The model under review builds one solid part; all positions refer to its coordinate system, in mm. A direction names the side the tool comes from. Give positions to 0.01 mm unless a question says otherwise; leave off trailing zeros. Order: outer loops, then holes, each group sorted by start corner. A loop starts at its lowest first (then second) coordinate and runs counter-clockwise, first axis right, second up.
```python
from build123d import *

# Parameters (mm, degrees)
BOSS_EXTRUDE1_DEPTH = 8
SKETCH4_W           = 10
SKETCH4_H           = 4
SKETCH4_W_2         = 4
SKETCH4_H_2         = 10
BOSS_EXTRUDE2_DEPTH = 14
SKETCH5_R           = 1
CUT_EXTRUDE1_DEPTH  = 16
SKETCH6_R           = 1
CUT_EXTRUDE2_DEPTH  = 16
FILLET1_R           = 2


with BuildPart() as part:
    # Sketch3 → Boss-Extrude1 (new body)
    with BuildSketch(Plane(origin=(0, 0, 0), x_dir=(1, 0, 0), z_dir=(0, 1, 0))):
        with BuildLine():
            Line((-40, 25), (40, 25))
            ThreePointArc((40, 25), (47.071067812, 22.071067812), (50, 15))
            Line((50, 15), (50, -15))
            ThreePointArc((50, -15), (47.071067812, -22.071067812), (40, -25))
            Line((40, -25), (-40, -25))
            ThreePointArc((-40, -25), (-47.071067812, -22.071067812), (-50, -15))
            Line((-50, -15), (-50, 15))
            ThreePointArc((-50, 15), (-47.071067812, 22.071067812), (-40, 25))
        make_face()
    extrude(amount=BOSS_EXTRUDE1_DEPTH)

    # Sketch4 → Boss-Extrude2 (add)
    with BuildSketch(Plane(origin=(0, 8, 0), x_dir=(1, 0, 0), z_dir=(0, 1, 0))):
        with Locations((-25, 20)):
            Rectangle(SKETCH4_W, SKETCH4_H)
        with Locations((-25, 8)):
            Rectangle(SKETCH4_W, SKETCH4_H)
        with Locations((-6, -9)):
            Rectangle(SKETCH4_W_2, SKETCH4_H_2)
        with Locations((6, -9)):
            Rectangle(SKETCH4_W_2, SKETCH4_H_2)
        with Locations((25, 8)):
            Rectangle(SKETCH4_W, SKETCH4_H)
        with Locations((25, 20)):
            Rectangle(SKETCH4_W, SKETCH4_H)
    extrude(amount=BOSS_EXTRUDE2_DEPTH)

    # Sketch5 → Cut-Extrude1 (cut)
    with BuildSketch(Plane.XY.offset(-6)):
        with Locations((-25, 18)):
            Circle(SKETCH5_R)
        with Locations((25, 18)):
            Circle(SKETCH5_R)
    extrude(amount=-CUT_EXTRUDE1_DEPTH, mode=Mode.SUBTRACT)

    # Sketch6 → Cut-Extrude2 (cut)
    with BuildSketch(Plane.ZY.offset(8)):
        with Locations((9, 18)):
            Circle(SKETCH6_R)
    extrude(amount=-CUT_EXTRUDE2_DEPTH, mode=Mode.SUBTRACT)

    # Fillet1
    fillet1_edges = [part.edges().sort_by_distance(p)[0] for p in [
        (47.071067812, 8, -22.071067812),
        (0, 8, -25),
        (-47.071067812, 8, -22.071067812),
        (-50, 8, 0),
        (-30, 22, -20),
        (-47.071067812, 8, 22.071067812),
        (-20, 22, -20),
        (0, 8, 25),
        (-30, 22, -8),
        (-20, 22, -8),
        (47.071067812, 8, 22.071067812),
        (-6, 22, 14),
        (-6, 22, 4),
        (6, 22, 4),
        (6, 22, 14),
        (30, 22, -8),
        (20, 22, -8),
        (30, 22, -20),
        (20, 22, -20),
        (50, 8, 0),
    ]]
    fillet(fillet1_edges, radius=FILLET1_R)


solid = part.part
```
Item 1: Take a section at A-A (z = 9). Give the boundary of the cut face in (x, y), and give its area (3 significant figures).
Values found:
outline: (-50, 0) - (50, 0) - (50, 6) arc R2 ccw to (48, 8) - (8, 8) - (8, 17) - (4, 17) - (4, 8) - (-4, 8) - (-4, 17) - (-8, 17) - (-8, 8) - (-48, 8) arc R2 ccw to (-50, 6) - close; (-8, 19) - (-4, 19) - (-4, 22) - (-8, 22) - close; (4, 19) - (8, 19) - (8, 22) - (4, 22) - close
area: 894 mm2
Item 2: For faces 1 (the flat face through (-30, 14, -8)), 2 (the flat face through (-25, 22, -8)), 3 (the flat face through (25, 15, -10)), 4 (the flat face through (20, 14, -8)), list the 3-axis set-ups (+Z, -Z, +X, -X, +Y, -Y) from which the entire face can be reached by the end or side of a thin tool; tool diameter is ignored.
Values found:
face 1: +Z, -Z, -X, +Y
face 2: +Z, -Z, +X, -X, +Y
face 3: +X, -X, +Y
face 4: +Z, -Z, +Y
Item 3: Draft analysis for pull direction Y (two halves, no side actions). For faces 5 (the flat face through (6, 22, 9)), 6 (the cylindrical face through (-25, 17, -8)), 7 (the flat face through (-6, 14, 4)), state which applies: released by +Y, released by -Y, zero draft, split by the parting line, or undercut.
Values found:
face 5: released by +Y
face 6: undercut
face 7: zero draft
Item 4: Take a section at C-C (y = 9.75). Give the boundary of the cut face in (x, z), and give its area (3 significant figures).
Values found:
outline: (-30, -22) - (-20, -22) - (-20, -18) - (-30, -18) - close; (-30, -10) - (-20, -10) - (-20, -6) - (-30, -6) - close; (-8, 4) - (-4, 4) - (-4, 14) - (-8, 14) - close; (4, 4) - (8, 4) - (8, 14) - (4, 14) - close; (20, -22) - (30, -22) - (30, -18) - (20, -18) - close; (20, -10) - (30, -10) - (30, -6) - (20, -6) - close
area: 240 mm2
Item 5: Take a section at B-B (x = -25). Give the boundary of the cut face in (y, z).
Values found:
outline: (0, -25) - (6, -25) arc R2 ccw to (8, -23) - (8, -22) - (17, -22) - (17, -18) - (8, -18) - (8, -10) - (17, -10) - (17, -6) - (8, -6) - (8, 23) arc R2 ccw to (6, 25) - (0, 25) - close; (19, -22) - (22, -22) - (22, -18) - (19, -18) - close; (19, -10) - (22, -10) - (22, -6) - (19, -6) - close
Item 6: For line 1 (Y direction, x = -25, z = -8); line 2 (Z direction, x = 21.5, y = 13.75); line 3 (Y direction, x = 39, z = 9.5), list the stretches that pass through material, from the lowest coordinate up.
Values found:
line 1: y = 0 to 17, 19 to 22
line 2: z = -22 to -18, -10 to -6
line 3: y = 0 to 8
Item 7: Clearance check with flat-ended pins moving along their axes: pin 1 Ø12 at (x, z) = (24.5, 17) entering from +Y; pin 2 Ø3 at (x, y) = (-3.5, 13.5) entering from -Z; pin 3 Ø3 at (x, y) = (-25, 18) entering from +Z. State where each tip first meets the part, or that it passes through.
Values found:
pin 1: stops at y = 8
pin 2: stops at z = 4
pin 3: stops at z = -6
Item 8: Take a section at D-D (z = -8). Give the boundary of the cut face in (x, y), and give its area (3 significant figures).
Values found:
outline: (-50, 0) - (50, 0) - (50, 6) arc R2 ccw to (48, 8) - (30, 8) - (30, 20) arc R2 ccw to (28, 22) - (22, 22) arc R2 ccw to (20, 20) - (20, 8) - (-20, 8) - (-20, 20) arc R2 ccw to (-22, 22) - (-28, 22) arc R2 ccw to (-30, 20) - (-30, 8) - (-48, 8) arc R2 ccw to (-50, 6) - close; hole circle Ø2 at (-25, 18); hole circle Ø2 at (25, 18)
area: 1,070 mm2
